```python
from build123d import *

# Parameters (mm, degrees)
SKETCH1_W           = 85.8
SKETCH1_H           = 92.5
BOSS_EXTRUDE1_DEPTH = 14.859
SKETCH2_W           = 85.8
SKETCH2_H           = 92.5
SKETCH2_R           = 1
BOSS_EXTRUDE2_DEPTH = 3.175
SKETCH4_W           = 85.8
SKETCH4_H           = 92.5
SKETCH4_W_2         = 75.8
SKETCH4_H_2         = 82.5
BOSS_EXTRUDE3_DEPTH = 4.5
CUT_EXTRUDE1_DEPTH  = 121.663419813
SKETCH5_W           = 14
SKETCH5_H           = 8
CUT_EXTRUDE2_DEPTH  = 121.663419813
SKETCH6_W           = 10
SKETCH6_H           = 6
CUT_EXTRUDE3_DEPTH  = 121.663419813
BOSS_EXTRUDE4_START = 1.9
SKETCH7_R           = 3.54
SKETCH7_R_2         = 1
BOSS_EXTRUDE4_DEPTH = 1.9
FILLET1_R           = 2.5
FILLET2_R           = 2.5
FILLET3_R           = 2.5
FILLET4_R           = 2.5
FILLET5_R           = 2.5
CUT_EXTRUDE4_DEPTH  = 1.5
CUT_EXTRUDE5_DEPTH  = 4
CUT_EXTRUDE7_DEPTH  = 73.9
SKETCH12_W          = 4.501
SKETCH12_H          = 4
BOSS_EXTRUDE8_DEPTH = 5


with BuildPart() as part:
    # Sketch1 → Boss-Extrude1 (new body)
    with BuildSketch(Plane(origin=(0, 0, 0), x_dir=(1, 0, 0), z_dir=(0, 1, 0))):
        with Locations((37.9, 41.25)):
            Rectangle(SKETCH1_W, SKETCH1_H)
        Polygon((5, 4), (5, 10), (0, 10), (0, 82.5), (70.8, 82.5), (70.8, 79), (75.8, 79), (75.8, 4), (59.9, 4), (59.9, 0), (52.9, 0), (52.9, 4), (41.4, 4), (41.4, 0), (34.4, 0), (34.4, 4), (22.9, 4), (22.9, 0), (15.9, 0), (15.9, 4), align=None, mode=Mode.SUBTRACT)
    extrude(amount=BOSS_EXTRUDE1_DEPTH)

    # Sketch2 → Boss-Extrude2 (add)
    with BuildSketch(Plane(origin=(0, 0, 0), x_dir=(1, 0, 0), z_dir=(0, 1, 0))):
        with Locations((37.9, 41.25)):
            Rectangle(SKETCH2_W, SKETCH2_H)
        with Locations(Location((3.5, 13.5, 0), (0, 0, 270))):
            Circle(SKETCH2_R, mode=Mode.SUBTRACT)
        with Locations(Location((19.4, 3.5, 0), (0, 0, 270))):
            Circle(SKETCH2_R, mode=Mode.SUBTRACT)
        with Locations(Location((37.9, 3.5, 0), (0, 0, 270))):
            Circle(SKETCH2_R, mode=Mode.SUBTRACT)
        with Locations(Location((56.4, 3.5, 0), (0, 0, 270))):
            Circle(SKETCH2_R, mode=Mode.SUBTRACT)
        with Locations(Location((30.3, 56.1, 0), (0, 0, 270))):
            Circle(SKETCH2_R, mode=Mode.SUBTRACT)
        with Locations(Location((71.8, 75.5, 0), (0, 0, 270))):
            Circle(SKETCH2_R, mode=Mode.SUBTRACT)
    extrude(amount=-BOSS_EXTRUDE2_DEPTH)

    # Sketch4 → Boss-Extrude3 (add)
    with BuildSketch(Plane(origin=(0, 14.859, 0), x_dir=(1, 0, 0), z_dir=(0, 1, 0))):
        with Locations((37.9, 41.25)):
            Rectangle(SKETCH4_W, SKETCH4_H)
        with Locations((37.9, 41.25)):
            Rectangle(SKETCH4_W_2, SKETCH4_H_2, mode=Mode.SUBTRACT)
    extrude(amount=BOSS_EXTRUDE3_DEPTH)

    # Sketch3 → Cut-Extrude1 (cut, through all)
    with BuildSketch(Plane(origin=(0, 0, 0), x_dir=(0, 0, -1), z_dir=(1, 0, 0))):
        with BuildLine():
            Line((60.6, 14.859), (60.6, 19.359))
            Line((60.6, 19.359), (51.6, 19.359))
            Line((51.6, 19.359), (51.6, 14.859))
            ThreePointArc((51.6, 14.859), (56.1, 10.359), (60.6, 14.859))
        make_face()
    extrude(amount=-CUT_EXTRUDE1_DEPTH, mode=Mode.SUBTRACT)

    # Sketch5 → Cut-Extrude2 (cut, through all)
    with BuildSketch(Plane.XY):
        with Locations((10.15, 20)):
            Rectangle(SKETCH5_W, SKETCH5_H)
        with Locations((28.65, 20)):
            Rectangle(SKETCH5_W, SKETCH5_H)
        with Locations((47.15, 20)):
            Rectangle(SKETCH5_W, SKETCH5_H)
        with Locations((65.65, 20)):
            Rectangle(SKETCH5_W, SKETCH5_H)
    extrude(amount=CUT_EXTRUDE2_DEPTH, mode=Mode.SUBTRACT)

    # Sketch6 → Cut-Extrude3 (cut, through all)
    with BuildSketch(Plane.XY):
        with Locations((59, 19.383)):
            Rectangle(SKETCH6_W, SKETCH6_H)
    extrude(amount=-CUT_EXTRUDE3_DEPTH, mode=Mode.SUBTRACT)

    # Sketch7 → Boss-Extrude4 (add)
    # profile 1 of 6: a face of its own
    with BuildSketch(Plane(origin=(0, 0, 0), x_dir=(1, 0, 0), z_dir=(0, 1, 0)).offset(BOSS_EXTRUDE4_START)):
        with Locations(Location((30.3, 56.1, 0), (0, 0, 90))):
            Circle(SKETCH7_R)
        with Locations(Location((30.3, 56.1, 0), (0, 0, 270))):
            Circle(SKETCH7_R_2, mode=Mode.SUBTRACT)
    # profile 2 of 6: a face of its own
    with BuildSketch(Plane(origin=(0, 0, 0), x_dir=(1, 0, 0), z_dir=(0, 1, 0)).offset(BOSS_EXTRUDE4_START)):
        with BuildLine():
            Line((0, 13.5), (0, 10))
            Line((0, 10), (3.5, 10))
            ThreePointArc((3.5, 10), (5.974873734, 15.974873734), (0, 13.5))
        make_face()
        with Locations(Location((3.5, 13.5, 0), (0, 0, 270))):
            Circle(SKETCH7_R_2, mode=Mode.SUBTRACT)
    # profile 3 of 6: a face of its own
    with BuildSketch(Plane(origin=(0, 0, 0), x_dir=(1, 0, 0), z_dir=(0, 1, 0)).offset(BOSS_EXTRUDE4_START)):
        with BuildLine():
            Line((15.9, 3.5), (15.9, 0))
            Line((15.9, 0), (22.9, 0))
            Line((22.9, 0), (22.9, 3.5))
            ThreePointArc((22.9, 3.5), (19.4, 7), (15.9, 3.5))
        make_face()
        with Locations(Location((19.4, 3.5, 0), (0, 0, 270))):
            Circle(SKETCH7_R_2, mode=Mode.SUBTRACT)
    # profile 4 of 6: a face of its own
    with BuildSketch(Plane(origin=(0, 0, 0), x_dir=(1, 0, 0), z_dir=(0, 1, 0)).offset(BOSS_EXTRUDE4_START)):
        with BuildLine():
            Line((34.4, 3.5), (34.4, 0))
            Line((34.4, 0), (41.4, 0))
            Line((41.4, 0), (41.4, 3.5))
            ThreePointArc((41.4, 3.5), (37.9, 7), (34.4, 3.5))
        make_face()
        with Locations(Location((37.9, 3.5, 0), (0, 0, 270))):
            Circle(SKETCH7_R_2, mode=Mode.SUBTRACT)
    # profile 5 of 6: a face of its own
    with BuildSketch(Plane(origin=(0, 0, 0), x_dir=(1, 0, 0), z_dir=(0, 1, 0)).offset(BOSS_EXTRUDE4_START)):
        with BuildLine():
            Line((52.9, 3.5), (52.9, 0))
            Line((52.9, 0), (59.9, 0))
            Line((59.9, 0), (59.9, 3.5))
            ThreePointArc((59.9, 3.5), (56.4, 7), (52.9, 3.5))
        make_face()
        with Locations(Location((56.4, 3.5, 0), (0, 0, 270))):
            Circle(SKETCH7_R_2, mode=Mode.SUBTRACT)
    # profile 6 of 6: a face of its own
    with BuildSketch(Plane(origin=(0, 0, 0), x_dir=(1, 0, 0), z_dir=(0, 1, 0)).offset(BOSS_EXTRUDE4_START)):
        with BuildLine():
            Line((75.8, 79), (69.863508327, 79))
            ThreePointArc((69.863508327, 79), (69.768493994, 72.054280431), (75.8, 75.5))
            Line((75.8, 75.5), (75.8, 79))
        make_face()
        with Locations(Location((71.8, 75.5, 0), (0, 0, 270))):
            Circle(SKETCH7_R_2, mode=Mode.SUBTRACT)
    extrude(amount=-BOSS_EXTRUDE4_DEPTH)

    # Fillet1
    fillet1_edges = [part.edges().sort_by_distance(p)[0] for p in [
        (-5, 8.092, 5),
    ]]
    fillet(fillet1_edges, radius=FILLET1_R)

    # Fillet2
    fillet2_edges = [part.edges().sort_by_distance(p)[0] for p in [
        (80.8, 8.092, 5),
    ]]
    fillet(fillet2_edges, radius=FILLET2_R)

    # Fillet3
    fillet3_edges = [part.edges().sort_by_distance(p)[0] for p in [
        (80.8, 8.092, -87.5),
    ]]
    fillet(fillet3_edges, radius=FILLET3_R)

    # Fillet4
    fillet4_edges = [part.edges().sort_by_distance(p)[0] for p in [
        (-5, 8.092, -87.5),
    ]]
    fillet(fillet4_edges, radius=FILLET4_R)

    # Fillet5
    fillet5_edges = [part.edges().sort_by_distance(p)[0] for p in [
        (37.9, -3.175, 5),
        (-4.267766953, -3.175, 4.267766953),
        (80.8, -3.175, -41.25),
        (80.067766953, -3.175, 4.267766953),
        (37.9, -3.175, -87.5),
        (80.067766953, -3.175, -86.767766953),
        (-5, -3.175, -41.25),
        (-4.267766953, -3.175, -86.767766953),
    ]]
    fillet(fillet5_edges, radius=FILLET5_R)

    # Sketch8 → Cut-Extrude4 (cut)
    with BuildSketch(Plane(origin=(0, 0, 0), x_dir=(0, 0, -1), z_dir=(1, 0, 0))):
        with BuildLine():
            Line((62.45, 14.855), (62.45, 21.205))
            Line((62.45, 21.205), (49.75, 21.205))
            Line((49.75, 21.205), (49.75, 14.855))
            ThreePointArc((49.75, 14.855), (56.1, 8.505), (62.45, 14.855))
        make_face()
    extrude(amount=-CUT_EXTRUDE4_DEPTH, mode=Mode.SUBTRACT)

    # Sketch9 → Cut-Extrude5 (cut)
    with BuildSketch(Plane(origin=(0, 19.359, 0), x_dir=(1, 0, 0), z_dir=(0, 1, 0))):
        Polygon((3.15, -1.8), (3.15, -3.2), (1.9, -2.5), align=None)
        Polygon((17.15, -1.8), (17.15, -3.2), (18.4, -2.5), align=None)
        Polygon((21.65, -1.8), (21.65, -3.2), (20.4, -2.5), align=None)
        Polygon((35.65, -1.8), (36.9, -2.5), (35.65, -3.2), align=None)
        Polygon((40.15, -1.8), (38.9, -2.5), (40.15, -3.2), align=None)
        Polygon((54.15, -1.8), (54.15, -3.2), (55.4, -2.5), align=None)
        Polygon((58.65, -1.8), (58.65, -3.2), (57.4, -2.5), align=None)
        Polygon((72.65, -1.8), (72.65, -3.2), (73.9, -2.5), align=None)
    extrude(amount=-CUT_EXTRUDE5_DEPTH, mode=Mode.SUBTRACT)

    # Sketch10 → Cut-Extrude7 (cut)
    with BuildSketch(Plane(origin=(0, 0, 0), x_dir=(0, 0, -1), z_dir=(1, 0, 0))):
        Polygon((-3.2, 16), (-1.8, 16), (-2.5, 14.7), align=None)
    extrude(amount=CUT_EXTRUDE7_DEPTH, mode=Mode.SUBTRACT)

    # Sketch12 → Boss-Extrude8 (add)
    with BuildSketch(Plane.XY):
        with Locations((0.8995, 14)):
            Rectangle(SKETCH12_W, SKETCH12_H)
        with Locations((19.3995, 14)):
            Rectangle(SKETCH12_W, SKETCH12_H)
        with Locations((37.8995, 14)):
            Rectangle(SKETCH12_W, SKETCH12_H)
        with Locations((56.3995, 14)):
            Rectangle(SKETCH12_W, SKETCH12_H)
        with Locations((74.9005, 14)):
            Rectangle(SKETCH12_W, SKETCH12_H)
    extrude(amount=BOSS_EXTRUDE8_DEPTH)


solid = part.part
```
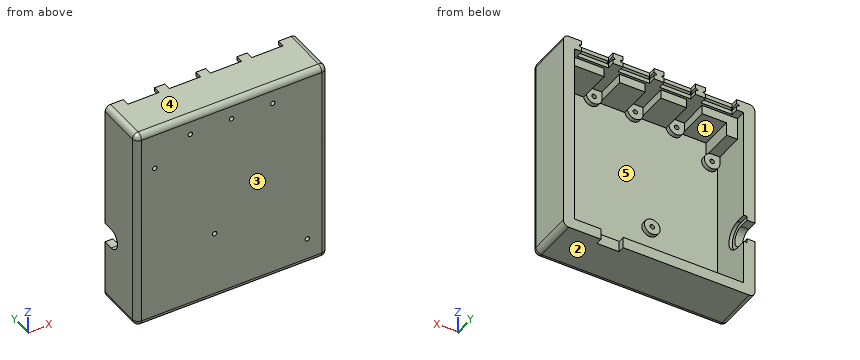
The model under review builds one solid part; all positions refer to its coordinate system, in mm. Face numbers are marked on the shaded views. A direction names the side the tool comes from. Give positions to 0.01 mm unless a question says otherwise; leave off trailing zeros. Loops run counter-clockwise (first coordinate to the right, second up) from the corner with the lowest first, then second, coordinate; pieces in that order, holes last. Notation, with made-up numbers: (9, 3) - (44, 3) arc R31 cw to (44, 37) - close; hole circle Ø3 at (80, -28.5). An arc over 180 degrees is marked (long way). Answer as a JSON object with one key per item and string values.
Q1. Mouldability with a two-part tool opening along Z and no side actions: class the marked faces 1, 2 and 3 as +Z half, -Z half, draft (parallel to the pull), parting line (faces both ways), or undercut.
Worked out:
{"face 1": "undercut", "face 2": "-Z half", "face 3": "draft"}
Q2. Insertion check: pin 1 (0.9 mm diameter, centred on y = 18.5, z = 4, fed in from +X); pin 2 (12 mm diameter, centred on x = 46.5, z = -36.5, fed in from +Y); pin 3 (11 mm diameter, centred on x = 12, z = -6.5, fed in from +Y). Each pin has a flat end and moves straight along its axis. Give the tip position at first contact, or say it passes through.
Worked out:
{"pin 1": "stops at x = 80.57", "pin 2": "stops at y = 0", "pin 3": "stops at y = 14.86"}
Q3. To check wall thickness, follow line 1 along X through (y, z) = (0.1, -56.1); line 2 along Z through (x, y) = (59, 13.5); line 3 along X through (y, z) = (12, -46). State the ranges of each line that lie inside material, in increasing order.
Worked out:
{"line 1": "x = -5 to 0, 26.76 to 29.3, 31.3 to 33.84, 75.8 to 80.8", "line 2": "z = -87.5 to -82.5, 0 to 5", "line 3": "x = -5 to 0, 75.8 to 80.8"}
Q4. Add section B-B on z = -28.5. State the section outline as (x, y) points (3 decimals).
Worked out:
{"outline": "(-5, -0.675) arc R2.5 ccw to (-2.5, -3.175) - (78.3, -3.175) arc R2.5 ccw to (80.8, -0.675) - (80.8, 19.359) - (75.8, 19.359) - (75.8, 0) - (0, 0) - (0, 19.359) - (-5, 19.359) - close"}
Q5. Add section A-A on x = 9.5. State the section outline as (y, z) points (3 decimals), plus the area to 3 significant figures.
Worked out:
{"outline": "(-3.175, -85) arc R2.5 ccw to (-0.675, -87.5) - (19.359, -87.5) - (19.359, -82.5) - (0, -82.5) - (0, -4) - (14.859, -4) - (14.859, 0) - (16, 0) - (16, 1.8) - (14.7, 2.5) - (16, 3.2) - (16, 5) - (-0.675, 5) arc R2.5 ccw to (-3.175, 2.5) - close", "area": "526 mm^2"}
Q6. For the marked faces 4 and 5, list the 3-axis set-ups (+Z, -Z, +X, -X, +Y, -Y) from which the entire face can be reached by the end or side of a thin tool; tool diameter is ignored.
Worked out:
{"face 4": "+Z, +X, -X, +Y, -Y", "face 5": "+Y"}
